from build123d import *

# Parameters (mm, degrees)
F0_R     = 2.15
F0_R_2   = 1.675
F0_W     = 2.5
F0_H     = 5.8
F1_DEPTH = 7
F2_DEPTH = 12
F3_R     = 2


with BuildPart() as f1:
    # F0 (on Top) → F1 (new body)
    with BuildSketch(Plane.XY):
        Polygon((-10, 7.1), (-10, 0), (10, 0), (10, 7.1), (7.5, 7.1), (7.5, 12.9), (10, 12.9), (10, 55), (-10, 55), (-10, 12.9), (-7.5, 12.9), (-7.5, 7.1), align=None)
        with Locations((0, 10)):
            Circle(F0_R, mode=Mode.SUBTRACT)
        with Locations((0, 30)):
            Circle(F0_R_2, mode=Mode.SUBTRACT)
        with Locations((0, 45)):
            Circle(F0_R_2, mode=Mode.SUBTRACT)
        with Locations((-8.75, 10)):
            Rectangle(F0_W, F0_H)
        with Locations((8.75, 10)):
            Rectangle(F0_W, F0_H)
    extrude(amount=F1_DEPTH)

    # F0 (on Top) → F2 (join)
    with BuildSketch(Plane.XY):
        with Locations((-8.75, 10)):
            Rectangle(F0_W, F0_H)
        with Locations((8.75, 10)):
            Rectangle(F0_W, F0_H)
    extrude(amount=F2_DEPTH)

    # F3
    f3_edges = [f1.edges().sort_by_distance(p)[0] for p in [
        (10, 0, 3.5),
        (-10, 0, 3.5),
        (10, 55, 3.5),
        (-10, 55, 3.5),
        (10, 27.5, 0),
        (0, 0, 0),
        (-10, 27.5, 0),
        (0, 55, 0),
    ]]
    fillet(f3_edges, radius=F3_R)


solid = f1.part
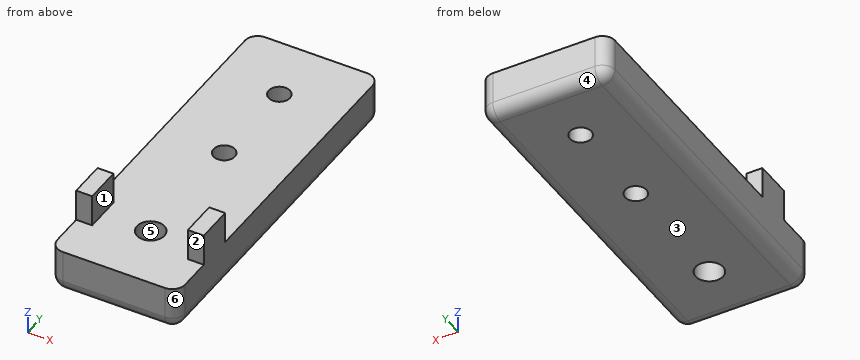
Geometry check sheet. Reference: the model listing, model coordinates, mm. Face numbers are marked on the shaded views. A direction names the side the tool comes from. Round coordinates to 2 decimals unless told otherwise and drop trailing zeros. Loops run counter-clockwise (first coordinate to the right, second up) from the corner with the lowest first, then second, coordinate; pieces in that order, holes last. Notation, with made-up numbers: (-22.5, 49.25) - (26.5, 49.25) arc R32 cw to (26.5, 80.25) - close; hole circle Ø2 at (80.25, 55.25). An arc over 180 degrees is marked (long way). One line per question, with ' | ' between items. Start each with the question number.
1. Depth check by flat-ended pin: pin 1 (2 mm diameter, centred on x = 1.5, y = 44.5, fed in from +Z); pin 2 (2 mm diameter, centred on x = -9, z = 9.5, fed in from +Y); pin 3 (2 mm diameter, centred on x = -8.5, z = 9.5, fed in from -Y). Enter the tip coordinate at first touch or a pass-through.
2. Cross-section at B-B on y = 30. Record the cut outline in (x, z) (3 decimals).
3. Scan lines: line 1 (Y direction, x = 0, z = 5) (3 decimals); line 2 (X direction, y = 8.5, z = 11); line 3 (Z direction, x = 0, y = 25.5). Record each from-to range of solid material in increasing order. Write a range as [from, to].
4. Cross-section at D-D on x = -6.5. Record the cut outline in (y, z), then the cut area to 3 significant figures.
5. Cross-section at A-A on x = 0. Record the cut outline in (y, z) (3 decimals), then the cut area to 3 significant figures.
6. Draft check along Y on the marked faces 4, 5 and 6. Enter one of: released by +Y, released by -Y, zero draft, split by the parting line, or undercut.
7. Tool access check on the marked faces 1, 2 and 3. Record the directions out of +Z, -Z, +X, -X, +Y, -Y that give a thin tool (end or side, any length) a straight path to the whole face; none if there is none.
8. Cross-section at C-C on z = 5.5. Record the cut outline in (x, y) (3 decimals).
Taken from the geometry:
1) pin 1: z = 7 | pin 2: y = 12.9 | pin 3: y = 7.1
2) outline: (-10, 2) arc R2 ccw to (-8, 0) - (-1.675, 0) - (-1.675, 7) - (-10, 7) - close; (1.675, 0) - (8, 0) arc R2 ccw to (10, 2) - (10, 7) - (1.675, 7) - close
3) line 1: [0, 7.85], [12.15, 28.325], [31.675, 43.325], [46.675, 55] | line 2: [-10, -7.5], [7.5, 10] | line 3: [0, 7]
4) outline: (0, 2) arc R2 ccw to (2, 0) - (53, 0) arc R2 ccw to (55, 2) - (55, 7) - (0, 7) - close | area: 383 mm²
5) outline: (0, 2) arc R2 ccw to (2, 0) - (7.85, 0) - (7.85, 7) - (0, 7) - close; (12.15, 0) - (28.325, 0) - (28.325, 7) - (12.15, 7) - close; (31.675, 0) - (43.325, 0) - (43.325, 7) - (31.675, 7) - close; (46.675, 0) - (53, 0) arc R2 ccw to (55, 2) - (55, 7) - (46.675, 7) - close | area: 306 mm²
6) face 4: released by +Y | face 5: undercut | face 6: released by -Y
7) face 1: +Z, +Y, -Y | face 2: +Z, +X, -X, -Y | face 3: -Z, +X, -X, +Y, -Y
8) outline: (-10, 2) arc R2 ccw to (-8, 0) - (8, 0) arc R2 ccw to (10, 2) - (10, 53) arc R2 ccw to (8, 55) - (-8, 55) arc R2 ccw to (-10, 53) - close; hole circle Ø4.3 at (0, 10); hole circle Ø3.35 at (0, 30); hole circle Ø3.35 at (0, 45)
